For this review, take the finished solid that the model builds, in its own axes (mm). Round coordinates to 2 decimals unless told otherwise and drop trailing zeros. Loops run counter-clockwise (first coordinate to the right, second up) from the corner with the lowest first, then second, coordinate; pieces in that order, holes last. Notation, with made-up numbers: M 39.25,-28 L 98.25,-28 A15 cw 98.25,-16 Z; hole C 14,-22 d4. An arc over 180 degrees is marked long. One line per question, with ' | ' between items. Start each with the question number.
1) We need section D-D (y = 1.2). State how many separate pieces and enclosed holes the cut face has, and give its area (3 significant figures).
2) For pin 1 Ø1 at (x, y) = (68, 1) entering from -Z; pin 2 Ø1 at (x, y) = (41, -0.5) entering from +Z, all flat-tipped, find the tip position at first contact; note any pin that passes through.
3) For probe 1 along X at (y, z) = (-1.05, 0); probe 2 along X at (y, z) = (-1, -86); probe 3 along X at (y, z) = (1.4, -85), list the stretches that pass through material, from the lowest coordinate up. Write a range as from..to.
4) We need section A-A (z = 0). Give the boundary of the cut face in (x, y).
5) We need section C-C (z = 30). Give the boundary of the cut face in (x, y), and give its area (3 significant figures).
6) Mouldability with a two-part tool opening along X and no side actions: class faces 1 (the face through (66.909, 0.028, -72.967)), 2 (the face through (81, -2, 7)), 3 (the face through (-67.752, -0.028, 56.126)) as pulls with the +X half, pulls with the -X half, needs draft (parallel to the pull), parting line crosses it, or undercut.
7) We need section B-B (x = 0). Give the boundary of the cut face in (y, z).
```python
from build123d import *

# Parameters (mm, degrees)
SKETCH1_R           = 99
SKETCH1_R_2         = 6
SKETCH1_R_3         = 81
BOSS_EXTRUDE1_DEPTH = 2


with BuildPart() as part:
    # Sketch1 → Boss-Extrude1 (new, symmetric)
    with BuildSketch(Plane(origin=(0, 0, 0), x_dir=(1, 0, 0), z_dir=(0, 1, 0))):
        with Locations(Location((0, 0, 0), (0, 0, 270))):
            Circle(SKETCH1_R)
        with Locations(Location((90, 0, 0), (0, 0, 270))):
            Circle(SKETCH1_R_2, mode=Mode.SUBTRACT)
        with Locations(Location((72.811529494, -52.900672706, 0), (0, 0, 270))):
            Circle(SKETCH1_R_2, mode=Mode.SUBTRACT)
        with Locations(Location((27.811529494, -85.595086467, 0), (0, 0, 270))):
            Circle(SKETCH1_R_2, mode=Mode.SUBTRACT)
        with Locations(Location((-27.811529494, -85.595086467, 0), (0, 0, 270))):
            Circle(SKETCH1_R_2, mode=Mode.SUBTRACT)
        with Locations(Location((-72.811529494, -52.900672706, 0), (0, 0, 270))):
            Circle(SKETCH1_R_2, mode=Mode.SUBTRACT)
        with Locations(Location((-90, 0, 0), (0, 0, 270))):
            Circle(SKETCH1_R_2, mode=Mode.SUBTRACT)
        with Locations(Location((-72.811529494, 52.900672706, 0), (0, 0, 270))):
            Circle(SKETCH1_R_2, mode=Mode.SUBTRACT)
        with Locations(Location((-27.811529494, 85.595086467, 0), (0, 0, 270))):
            Circle(SKETCH1_R_2, mode=Mode.SUBTRACT)
        with Locations(Location((27.811529494, 85.595086467, 0), (0, 0, 270))):
            Circle(SKETCH1_R_2, mode=Mode.SUBTRACT)
        with Locations(Location((72.811529494, 52.900672706, 0), (0, 0, 270))):
            Circle(SKETCH1_R_2, mode=Mode.SUBTRACT)
        with Locations(Location((0, 0, 0), (0, 0, 270))):
            Circle(SKETCH1_R_3, mode=Mode.SUBTRACT)
    extrude(amount=BOSS_EXTRUDE1_DEPTH, both=True)


solid = part.part
```
Answers below:
1) separate pieces: 1 | enclosed holes: 11 | area: 9,050 mm^2
2) pin 1: z = -72.42 | pin 2: z = 90.34
3) probe 1: -99..-96, -84..-81, 81..84, 96..99 | probe 2: -49.04..-33.8, -21.83..21.83, 33.8..49.04 | probe 3: -50.75..-33.78, -21.84..21.84, 33.78..50.75
4) outline: M -99,-2 L -96,-2 L -96,2 L -99,2 Z; M -84,-2 L -81,-2 L -81,2 L -84,2 Z; M 81,-2 L 84,-2 L 84,2 L 81,2 Z; M 96,-2 L 99,-2 L 99,2 L 96,2 Z
5) outline: M -94.35,-2 L -75.24,-2 L -75.24,2 L -94.35,2 Z; M 75.24,-2 L 94.35,-2 L 94.35,2 L 75.24,2 Z | area: 153 mm^2
6) face 1: parting line crosses it | face 2: needs draft | face 3: undercut
7) outline: M -2,-99 L 2,-99 L 2,-81 L -2,-81 Z; M -2,81 L 2,81 L 2,99 L -2,99 Z
